Here's how the part is built. I have some questions about the finished solid (model axes, mm). Face numbers are marked on the shaded views. Round coordinates to 2 decimals unless told otherwise and drop trailing zeros. Loops run counter-clockwise (first coordinate to the right, second up) from the corner with the lowest first, then second, coordinate; pieces in that order, holes last. Notation, with made-up numbers: M 49,34 L 81,34 A23 cw 81,62 Z; hole C -31,15.5 d11. An arc over 180 degrees is marked long. Write each question's results on one line, items separated by ' | '. Start each with the question number.
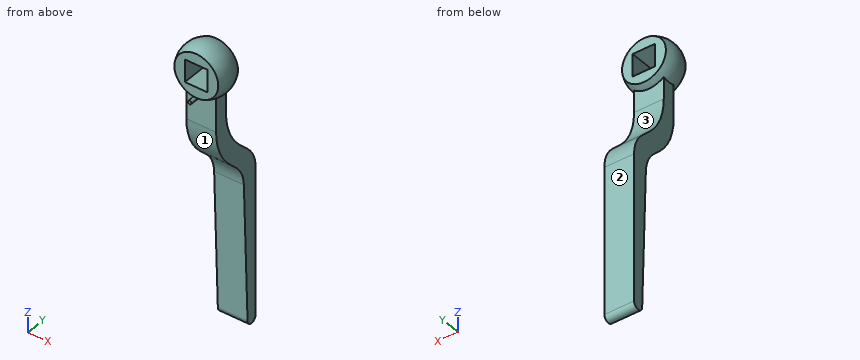
```python
from build123d import *

# Parameters (mm, degrees)
BOSS_EXTRUDE1_DEPTH     = 12.5
CUT_EXTRUDE1_DEPTH      = 219.987073
CUT_EXTRUDE1_DEPTH_BACK = 219.987073
CUT_EXTRUDE2_DEPTH      = 218.323119
CUT_EXTRUDE2_DEPTH_BACK = 218.323119
SKETCH4_W               = 19
SKETCH4_H               = 19
SKETCH6_R               = 1.5
BOSS_EXTRUDE2_DEPTH     = 7.5


with BuildPart() as part:
    # Sketch1 → Boss-Extrude1 (new, symmetric)
    with BuildSketch(Plane(origin=(0, 0, 0), x_dir=(0, 0, -1), z_dir=(1, 0, 0))):
        with BuildLine():
            Line((0, -5.5), (0, 5.5))
            Line((0, 5.5), (20, 5.5))
            ThreePointArc((20, 5.5), (39.516855, 9.382144), (56.062446, 20.437554))
            Line((56.062446, 20.437554), (65.630988, 30.006097))
            ThreePointArc((65.630988, 30.006097), (75.039265, 36.292506), (86.137085, 38.5))
            Line((86.137085, 38.5), (210, 38.5))
            ThreePointArc((210, 38.5), (214.500685, 34.077189), (210.157096, 29.5))
            Line((210.157096, 29.5), (93.053311, 25.410646))
            ThreePointArc((93.053311, 25.410646), (82.501674, 23.023054), (73.5593, 16.934408))
            Line((73.5593, 16.934408), (66.062446, 9.437554))
            ThreePointArc((66.062446, 9.437554), (49.516855, -1.617856), (30, -5.5))
            Line((30, -5.5), (0, -5.5))
        make_face()
    extrude(amount=BOSS_EXTRUDE1_DEPTH, both=True)

    # Sketch2 → Revolve2 (revolve)
    with BuildSketch(Plane(origin=(0, 0, 0), x_dir=(0, 0, -1), z_dir=(1, 0, 0))):
        with BuildLine():
            Line((-36.5, 0), (6.5, 0))
            ThreePointArc((6.5, 0), (-15, 21.5), (-36.5, 0))
        make_face()
    revolve(axis=Axis((0, 0, 36.5), (0, 0, -1)))

    # Sketch3 → Cut-Extrude1 (cut, two sides: drawn at the far end of the back side and taken through both)
    with BuildSketch(Plane(origin=(0, 0, 0), x_dir=(0, 0, -1), z_dir=(1, 0, 0)).offset(-CUT_EXTRUDE1_DEPTH_BACK)):
        with BuildLine():
            Line((-33.472953, 11), (3.472953, 11))
            ThreePointArc((3.472953, 11), (-15, 21.5), (-33.472953, 11))
        make_face()
        with BuildLine():
            Line((-33.472953, -11), (3.472953, -11))
            ThreePointArc((3.472953, -11), (-15, -21.5), (-33.472953, -11))
        make_face()
    extrude(amount=CUT_EXTRUDE1_DEPTH + CUT_EXTRUDE1_DEPTH_BACK, mode=Mode.SUBTRACT)

    # Sketch4 → Cut-Extrude2 (cut, two sides: drawn at the far end of the back side and taken through both)
    with BuildSketch(Plane(origin=(0, 11, 0), x_dir=(1, 0, 0), z_dir=(0, 1, 0)).offset(-CUT_EXTRUDE2_DEPTH_BACK)):
        with Locations((0, -15)):
            Rectangle(SKETCH4_W, SKETCH4_H)
    extrude(amount=CUT_EXTRUDE2_DEPTH + CUT_EXTRUDE2_DEPTH_BACK, mode=Mode.SUBTRACT)

    # Sketch6 → Boss-Extrude2 (add, symmetric)
    with BuildSketch(Plane.XZ.offset(5.5)):
        with Locations(Location((-4, -8, 0), (0, 0, 90))):
            Circle(SKETCH6_R)
    extrude(amount=BOSS_EXTRUDE2_DEPTH, both=True)


solid = part.part
```
1. For pin 1 (15 mm diameter, centred on y = -2, z = 11, fed in from +X); pin 2 (9.5 mm diameter, centred on y = 2.5, z = 18.5, fed in from -X); pin 3 (9.5 mm diameter, centred on x = -4.5, y = 2, fed in from +Z), each with a flat end and sliding along its axis, tell me the tip position at first contact or that it passes through.
2. I want a section at C-C on z = -122. List the corners of the cut face in (x, y) for me.
3. I want a section at B-B on x = -15.5. List the corners of the cut face in (y, z) for me, plus the area to 3 significant figures.
4. If we mould it in two halves opening along Z, with no side actions, what happens to the marked faces 1, 2 and 3? For each: released by +Z, released by -Z, zero draft, split by the parting line, or undercut.
5. I need wall thicknesses on line 1 along Z through (x, y) = (3, 0); line 2 along X through (y, z) = (-4.5, 21); line 3 along X through (y, z) = (29.5, -100). Which ranges of each line are inside material? Lowest first, please.
6. I want a section at A-A on y = 3. List the corners of the cut face in (x, z) for me, plus the area to 3 significant figures.
Outcome:
1) pin 1: x = 21.5 | pin 2: x = -21.5 | pin 3: z = 36.5
2) outline: M -12.5,26.42 L 12.5,26.42 L 12.5,38.5 L -12.5,38.5 Z
3) outline: M -11,4.95 A14.9 ccw 11,4.95 L 11,25.05 A14.9 ccw -11,25.05 Z | area: 590 mm2
4) face 1: released by -Z | face 2: zero draft | face 3: undercut
5) line 1: -53.04 to 5.5, 24.5 to 36.29 | line 2: -20.15 to -9.5, 9.5 to 20.15 | line 3: -12.5 to 12.5
6) outline: M -12.5,-58.19 L 12.5,-58.19 L 12.5,-2.23 A21.29 ccw long -12.5,-2.23 Z; hole M -9.5,5.5 L 9.5,5.5 L 9.5,24.5 L -9.5,24.5 Z | area: 2,390 mm2
